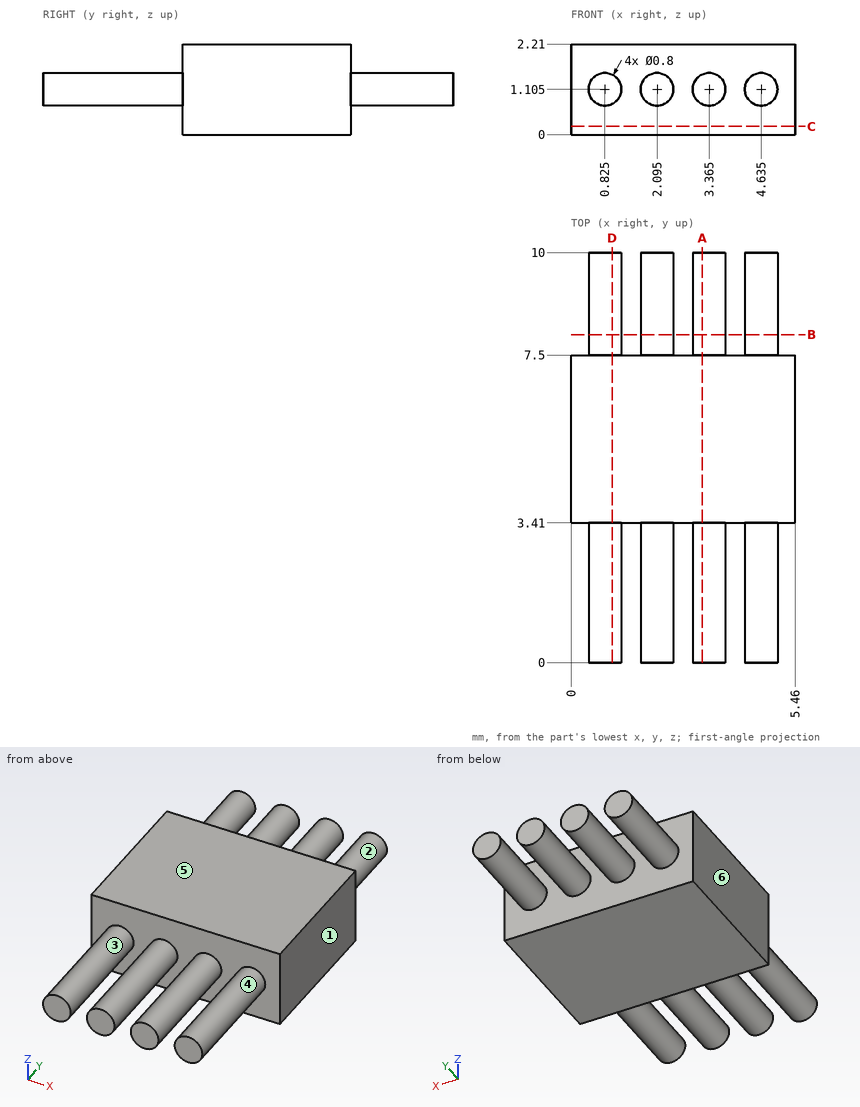
Can you work these out from the drawing? Everything is in mm from the part's minimum corner. A direction names the side the tool comes from. Give positions to 0.01 mm unless a question says otherwise; leave off trailing zeros. Order: outer loops, then holes, each group sorted by start corner. A loop starts at its lowest first (then second) coordinate and runs counter-clockwise, first axis right, second up. Notation, with made-up numbers: M 71.25,39 L 76.25,39 A16 ccw 76.25,67 Z; hole C -10,3.5 d5. An arc over 180 degrees is marked long. Write item = value, one per line. Start each with the question number.
Q1. I need wall thicknesses on probe 1 along Y at (x, z) = (3.4, 2.05); probe 2 along Z at (x, y) = (3.35, 8); probe 3 along Z at (x, y) = (1.1, 2.5). Which ranges of each line are inside material? Lowest first, please. Write a range as [from, to].
Q2. Suppose I cut it at A-A (x = 3.2). Write out the boundary of the cut face in (y, z).
Q3. Suppose I cut it at B-B (y = 8). Write out the boundary of the cut face in (x, z) (3 decimals), plus the area to 3 significant figures.
Q4. Suppose I cut it at C-C (z = 0.2). Write out the boundary of the cut face in (x, y).
Q5. For the marked faces 1, 2 and 3, which set-ups out of +Z, -Z, +X, -X, +Y, -Y let a thin tool reach every point of the face, with its end or its side?
Q6. We'd pull the mould along X, two halves only. Please class the marked faces 4, 5 and 6: pulls with the +X half, pulls with the -X half, needs draft (parallel to the pull), parting line crosses it, or undercut.
Q7. Suppose I cut it at D-D (x = 1). Write out the boundary of the cut face in (y, z).
Check result:
q1.probe_1 = [3.41, 7.5]
q1.probe_2 = [0.71, 1.5]
q1.probe_3 = [0.81, 1.4]
q2.outline = M 0,0.74 L 3.41,0.74 L 3.41,0 L 7.5,0 L 7.5,0.74 L 10,0.74 L 10,1.47 L 7.5,1.47 L 7.5,2.21 L 3.41,2.21 L 3.41,1.47 L 0,1.47 Z
q3.outline = C 0.825,1.105 d0.8; C 2.095,1.105 d0.8; C 3.365,1.105 d0.8; C 4.635,1.105 d0.8
q3.area = 2.01 mm2
q4.outline = M 0,3.41 L 5.46,3.41 L 5.46,7.5 L 0,7.5 Z
q5.face_1 = +Z, -Z, +X, +Y, -Y
q5.face_2 = +Y
q5.face_3 = -Y
q6.face_4 = undercut
q6.face_5 = needs draft
q6.face_6 = pulls with the -X half
q7.outline = M 0,0.75 L 3.41,0.75 L 3.41,0 L 7.5,0 L 7.5,0.75 L 10,0.75 L 10,1.46 L 7.5,1.46 L 7.5,2.21 L 3.41,2.21 L 3.41,1.46 L 0,1.46 Z
